```python
from build123d import *

# Parameters (mm, degrees)
SKETCH1_W                = 25
SKETCH1_H                = 25
BOSS_EXTRUDE1_DEPTH      = 10
BOSS_EXTRUDE2_DEPTH      = 12.5
BOSS_EXTRUDE2_DEPTH_BACK = 12.5
SKETCH2_R                = 6.5
SKETCH2_R_2              = 2.5
SKETCH3_W                = 25.519828657
SKETCH3_H                = 10
SKETCH3_W_2              = 24.900390406
SKETCH3_H_2              = 11.424636542
SKETCH3_H_3              = 9.385874126
CUT_EXTRUDE1_DEPTH       = 22.5


with BuildPart() as part:
    # Sketch1 → Boss-Extrude1 (new body)
    with BuildSketch(Plane(origin=(0, 0, 0), x_dir=(1, 0, 0), z_dir=(0, 1, 0))):
        Rectangle(SKETCH1_W, SKETCH1_H)
    extrude(amount=-BOSS_EXTRUDE1_DEPTH)

    # Sketch2 → Boss-Extrude2 (add, two sides: drawn at the far end of the back side and taken through both)
    # profile 1 of 4: a face of its own
    with BuildSketch(Plane.XY.offset(-BOSS_EXTRUDE2_DEPTH_BACK)):
        with Locations((-16.5, 6.5)):
            Circle(SKETCH2_R)
        with Locations((-16.5, 6.5)):
            Circle(SKETCH2_R_2, mode=Mode.SUBTRACT)
    # profile 2 of 4: a face of its own
    with BuildSketch(Plane.XY.offset(-BOSS_EXTRUDE2_DEPTH_BACK)):
        with BuildLine():
            ThreePointArc((-10, 6.5), (-11.903805922, 1.903805922), (-16.5, 0))
            Line((-16.5, 0), (-12.5, 0))
            Line((-12.5, 0), (0, 0))
            Line((0, 0), (-10, 6.5))
        make_face()
    # profile 3 of 4: a face of its own
    with BuildSketch(Plane.XY.offset(-BOSS_EXTRUDE2_DEPTH_BACK)):
        with BuildLine():
            Line((10, 6.5), (0, 0))
            Line((0, 0), (12.5, 0))
            Line((12.5, 0), (16.5, 0))
            ThreePointArc((16.5, 0), (11.903805922, 1.903805922), (10, 6.5))
        make_face()
    # profile 4 of 4: a face of its own
    with BuildSketch(Plane.XY.offset(-BOSS_EXTRUDE2_DEPTH_BACK)):
        with Locations((16.5, 6.5)):
            Circle(SKETCH2_R)
        with Locations((16.5, 6.5)):
            Circle(SKETCH2_R_2, mode=Mode.SUBTRACT)
    extrude(amount=BOSS_EXTRUDE2_DEPTH + BOSS_EXTRUDE2_DEPTH_BACK)

    # Sketch3 → Cut-Extrude1 (cut)
    with BuildSketch(Plane(origin=(0, 0, 0), x_dir=(1, 0, 0), z_dir=(0, 1, 0))):
        with Locations((-12.759914329, 0)):
            Rectangle(SKETCH3_W, SKETCH3_H)
        with Locations((12.450195203, 10.712318271)):
            Rectangle(SKETCH3_W_2, SKETCH3_H_2)
        with Locations((12.450195203, -9.692937063)):
            Rectangle(SKETCH3_W_2, SKETCH3_H_3)
    extrude(amount=CUT_EXTRUDE1_DEPTH, mode=Mode.SUBTRACT)


solid = part.part
```
For this review, take the finished solid that the model builds, in its own axes (mm). A direction names the side the tool comes from. Coordinates: 2 decimals unless noted, no trailing zeros. Write each loop counter-clockwise with the first axis right and the second up, starting at its lowest first coordinate (ties: lowest second). Pieces come first, ordered by that corner, then holes. Notation, with made-up numbers: (-18, 8.25) -> (3, 8.25) arc R28 ccw to (3, 31.25) -> close; hole circle Ø2 at (59, 86.25). An arc over 180 degrees is marked (long way). Put each result on its own line as item: value.
Q1. Take a section at D-D, the plane x = -15. State the section outline as (y, z) points, then the cut area to 3 significant figures.
From the geometry:
outline: (0, -12.5) -> (4.5, -12.5) -> (4.5, -5) -> (0, -5) -> close; (0, 5) -> (4.5, 5) -> (4.5, 12.5) -> (0, 12.5) -> close; (8.5, -12.5) -> (12.82, -12.5) -> (12.82, -5) -> (8.5, -5) -> close; (8.5, 5) -> (12.82, 5) -> (12.82, 12.5) -> (8.5, 12.5) -> close
area: 132 mm2
Q2. Wall thickness on L1, parallel to Y at x = -16.5, z = -10.25; L2, parallel to Z at x = -11.5, y = 1; L3, parallel to X at y = -1.75, z = 11.75: over which ranges is each line inside the solid? List them lowest first.
From the geometry:
L1: y = 0 to 4, 9 to 13
L2: z = -12.5 to -5, 5 to 12.5
L3: x = -12.5 to 12.5
Q3. Clearance check with flat-ended pins moving along their axes: pin 1 Ø2 at (x, z) = (4, -10.5) entering from +Y; pin 2 Ø11 at (y, z) = (-7, -4) entering from +X; pin 3 Ø8 at (x, z) = (5, 8.5) entering from +Y. State where each tip first meets the part, or that it passes through.
From the geometry:
pin 1: stops at y = 0
pin 2: stops at x = 12.5
pin 3: stops at y = 4.51
Q4. Take a section at C-C, the plane y = 7. State the section outline as (x, z) points, then the cut area to 3 significant figures.
From the geometry:
outline: (-22.98, -12.5) -> (-18.95, -12.5) -> (-18.95, -5) -> (-22.98, -5) -> close; (-22.98, 5) -> (-18.95, 5) -> (-18.95, 12.5) -> (-22.98, 12.5) -> close; (-14.05, -12.5) -> (-10.02, -12.5) -> (-10.02, -5) -> (-14.05, -5) -> close; (-14.05, 5) -> (-10.02, 5) -> (-10.02, 12.5) -> (-14.05, 12.5) -> close; (10.02, -5) -> (14.05, -5) -> (14.05, 5) -> (10.02, 5) -> close; (18.95, -5) -> (22.98, -5) -> (22.98, 5) -> (18.95, 5) -> close
area: 202 mm2
Q5. Take a section at A-A, the plane z = 7. State the section outline as (x, y) points, then the cut area to 3 significant figures.
From the geometry:
outline: (-16.5, 0) -> (-12.5, 0) -> (-12.5, -10) -> (12.5, -10) -> (12.5, 0) -> (0, 0) -> (-10, 6.5) arc R6.5 ccw (long way) to start; hole circle Ø5 at (-16.5, 6.5)
area: 405 mm2
Q6. Take a section at B-B, the plane x = -8. State the section outline as (y, z) points.
From the geometry:
outline: (-10, -12.5) -> (5.2, -12.5) -> (5.2, -5) -> (0, -5) -> (0, 5) -> (5.2, 5) -> (5.2, 12.5) -> (-10, 12.5) -> close
Q7. The part is to be moulded in two halves that separate along Z. For faces 1 (the flat face through (14, 5, 5)), 2 (the flat face through (-14, 5, -5)), 3 (the flat face through (6, 0, 9)), say which applies: +Z half, -Z half, draft (parallel to the pull), parting line (faces both ways), or undercut.
From the geometry:
face 1: +Z half
face 2: undercut
face 3: draft
Q8. Tool access review of faces 4 (the flat face through (-14, 5, 5)), 5 (the flat face through (0, -10, 0)), 6 (the flat face through (6, 0, -9)), 7 (the flat face through (-12.5, -5, 0)), 8 (the flat face through (14, 0, 0)): name each direction out of +Z, -Z, +X, -X, +Y, -Y from which nothing blocks a thin tool from reaching the whole face with its end or side.
From the geometry:
face 4: -X, +Y
face 5: +Z, -Z, +X, -X, -Y
face 6: -Z, +X, +Y
face 7: +Z, -Z, -X, -Y
face 8: +Z, -Z, +X, -Y
